The model under review builds one solid part; all positions refer to its coordinate system, in mm. Face numbers are marked on the shaded views. A direction names the side the tool comes from. Round coordinates to 2 decimals unless told otherwise and drop trailing zeros. Order: outer loops, then holes, each group sorted by start corner. A loop starts at its lowest first (then second) coordinate and runs counter-clockwise, first axis right, second up. Notation, with made-up numbers: (-9.5, 17.5) -> (8.5, 17.5) arc R15 cw to (8.5, 26.5) -> close; hole circle Ø6 at (71.25, 54). An arc over 180 degrees is marked (long way). Use a Markdown table: item, result. Add a question column.
Autodesk Fusion 360 part; units mm, degrees
sketch "Sketch1" plane through (0, 0, 0) normal (0, 1, 0) x (1, 0, 0)
  circle A0 centre (0, 0) radius 2.75
  circle A1 centre (0, 0) radius 6.75
  dimension "d1" = 5.5
  dimension "d2" = 4
extrude "Extrude1" add sketch "Sketch1" along normal blind 12
ref_plane "WorkPlane1" through (3, 0, 0) normal (1, 0, 0) x (0, 1, 0)
sketch "Sketch2" plane through (3, 0, 0) normal (1, 0, 0) x (0, 1, 0)
  line L0 (12, -6.75) -> (12, 6.75)
  line L1 (0, -6.75) -> (0, 6.75)
  circle A0 centre (6, 0) radius 4.6
  circle A1 centre (6, 0) radius 6
  dimension "d6" = 9.2
  dimension "d7" = 6
  dimension "d8" = 12
  dimension "d9" = 1.4
extrude "Extrude2" add sketch "Sketch2" along normal blind 8
ref_plane "WorkPlane2" through (2.75, 6.403, 0) normal (-1, 0, 0) x (0, 0, -1)
sketch "Sketch3" plane through (2.75, 6.403, 0) normal (-1, 0, 0) x (0, -1, 0)
  line L0 (-5.597, -2.75) -> (-5.597, 2.75)
  line L1 (6.403, -2.75) -> (6.403, 2.75)
  line L2 (6.403, -2.75) -> (6.403, 2.75)
  line L3 (-5.597, -2.75) -> (-5.597, 2.75)
  circle A0 centre (0.403, 0) radius 3.5
  point P0 (0.403, 0)
  dimension "d13" = 6
  dimension "d14" = 12
  dimension "d20" = 7
hole "Hole1" at (2.75, 6, 0) direction (1, 0, 0) diameter 3 depth 10 tip angle 118 counterbore diameter 7 counterbore depth 2
extrude "Extrude3" cut sketch "Sketch3" along normal blind 14.5
sketch "Sketch4" plane through (0, 0, 0) normal (0, 1, 0) x (1, 0, 0)
hole "Hole2" at (0, 0, 0) direction (0, -1, 0) diameter 5.5 depth 25.5 tip angle 118 countersink diameter 11.2 countersink angle 90
equation "d1 = 5 mm + 0.5 mm"
equation "d6 = 9 mm + 0.2 mm"
equation "d7 = d8 / 2"
equation "d13 = d14 / 2"
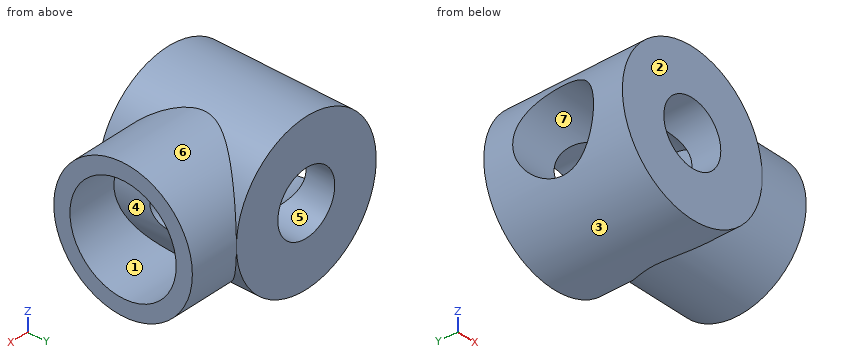
Q1. Machinability: for the marked faces 5, 6 and 7, which of the approach directions +Z, -Z, +X, -X, +Y, -Y give a long, thin tool a straight path to every point of the face, cutting with its end or side? Answer none if there is none.
Q2. Mouldability with a two-part tool opening along Z and no side actions: class the marked faces 1, 2, 3 and 4 as pulls with the +Z half, pulls with the -Z half, needs draft (parallel to the pull), parting line crosses it, or undercut.
Q3. Wall thickness on line 1 (Z direction, x = 7.25, y = 6); line 2 (Y direction, x = 9, z = 0); line 3 (Y direction, x = 5.3, z = 0): over which ranges is each line inside the solid? List them lowest first. Write a range as [from, to].
Q4. Add section A-A (x = 0). Write out the cut boundary in (y, z).
Q5. Insertion check: pin 1 (2 mm diameter, centred on y = 5, z = -1.5, fed in from -X); pin 2 (3 mm diameter, centred on x = 4.5, y = 5.5, fed in from -Z); pin 3 (1 mm diameter, centred on x = 6.5, y = 8.5, fed in from -Z). Each pin has a flat end and moves straight along its axis. Give the tip position at first contact, or say it passes through.
Q6. Add section C-C (z = -5). Write out the cut boundary in (x, y).
Report:
| question | item | result |
|---|---|---|
| 1 | face 5 | +Y, -Y |
| 1 | face 6 | +X |
| 1 | face 7 | -X |
| 2 | face 1 | undercut |
| 2 | face 2 | needs draft |
| 2 | face 3 | parting line crosses it |
| 2 | face 4 | undercut |
| 3 | line 1 | z = [-6, -4.6], [4.6, 6] |
| 3 | line 2 | y = [0, 1.4], [10.6, 12] |
| 3 | line 3 | y = [0, 4.5], [7.5, 12] |
| 4 | outline | (0, -6.75) -> (12, -6.75) -> (12, -2.75) -> (8.17, -2.75) arc R3.5 cw to (3.83, -2.75) -> (0, -2.75) -> close; (0, 2.75) -> (3.83, 2.75) arc R3.5 cw to (8.17, 2.75) -> (12, 2.75) -> (12, 6.75) -> (0, 6.75) -> close |
| 5 | pin 1 | stops at x = 4.75 |
| 5 | pin 2 | stops at z = -6.05 |
| 5 | pin 3 | stops at z = -5.66 |
| 6 | outline | (-4.53, 0) -> (4.53, 0) -> (4.53, 2.68) -> (11, 2.68) -> (11, 9.32) -> (4.53, 9.32) -> (4.53, 12) -> (-4.53, 12) -> close |
